Model file for the job. Use its own axes, mm. A direction names the side the tool comes from. Give positions to 0.01 mm unless a question says otherwise; leave off trailing zeros. Loops run counter-clockwise (first coordinate to the right, second up) from the corner with the lowest first, then second, coordinate; pieces in that order, holes last. Notation, with made-up numbers: M 33.5,-23 L 82.5,-23 A23 ccw 82.5,3 Z; hole C 52,-4.5 d10. An arc over 180 degrees is marked long. Answer in a Markdown table with one row per item.
```python
from build123d import *

# Parameters (mm, degrees)
BOSS_EXTRUDE1_DEPTH = 40
CUT_EXTRUDE1_REACH  = 97.146
SKETCH2_W           = 12.7
SKETCH2_H           = 36.204742391
CUT_EXTRUDE2_REACH  = 87.131
SKETCH3_W           = 56.49525371
SKETCH3_H           = 18.41246495
BOSS_EXTRUDE3_DEPTH = 2


with BuildPart() as part:
    # Sketch1 → Boss-Extrude1 (new body)
    with BuildSketch(Plane.XY):
        Polygon((-19.897004387, 33.25), (-35, 20.138954141), (-35, -20.138954141), (-19.897004387, -33.25), (19.897004387, -33.25), (35, -20.138954141), (35, 20.138954141), (19.897004387, 33.25), align=None)
        Polygon((19.15, 31.25), (33, 19.226690863), (33, -19.226690863), (19.15, -31.25), (-19.15, -31.25), (-33, -19.226690863), (-33, 19.226690863), (-19.15, 31.25), align=None, mode=Mode.SUBTRACT)
    extrude(amount=BOSS_EXTRUDE1_DEPTH)

    # Sketch2 → Cut-Extrude1 (cut, up to next)
    with BuildSketch(Plane(origin=(25.010799593, -28.810668547, 0), x_dir=(0.7551497806531032, 0.6555522929405175, 0), z_dir=(0.6555522929405175, -0.7551497806531032, 0)), mode=Mode.PRIVATE) as cut_extrude1_sk1:
        with Locations((6.878104758, 33.102371196)):
            Rectangle(SKETCH2_W, SKETCH2_H)
    cut_extrude1_tool1 = extrude(cut_extrude1_sk1.sketch, amount=-CUT_EXTRUDE1_REACH, mode=Mode.PRIVATE) & part.part
    cut_extrude1 = cut_extrude1_tool1.solids().sort_by_distance((30.204799, -24.301711, 33.102371))[0]
    add(cut_extrude1, mode=Mode.SUBTRACT)

    # Mirror1: Cut-Extrude1 across plane
    add(cut_extrude1.mirror(Plane(origin=(0, 0, 0), x_dir=(0, 0, 1), z_dir=(1, 0, 0))), mode=Mode.SUBTRACT)

    # Sketch3 → Cut-Extrude2 (cut, up to next)
    with BuildSketch(Plane.XZ.offset(33.25), mode=Mode.PRIVATE) as cut_extrude2_sk1:
        with Locations((-0.191025239, 37.206232475)):
            Rectangle(SKETCH3_W, SKETCH3_H)
    cut_extrude2_tool1 = extrude(cut_extrude2_sk1.sketch, amount=-CUT_EXTRUDE2_REACH, mode=Mode.PRIVATE) & part.part
    add(cut_extrude2_tool1.solids().sort_by_distance((-0.191025, -33.25, 37.206232))[0], mode=Mode.SUBTRACT)

    # Sketch4 → Boss-Extrude3 (add)
    with BuildSketch(Plane.XY):
        Polygon((19.15, 31.25), (33, 19.226690863), (33, -19.226690863), (19.15, -31.25), (-19.15, -31.25), (-33, -19.226690863), (-33, 19.226690863), (-19.15, 31.25), align=None)
    extrude(amount=BOSS_EXTRUDE3_DEPTH)


solid = part.part
```
Q1. Probe probe 1 along Y at (x, z) = (-13, 18.5); probe 2 along X at (y, z) = (11, 37.5); probe 3 along Z at (x, y) = (19, 17). List the from-to ranges inside material, lowest first.
Reported:
| item | result |
|---|---|
| probe 1 | -33.25 to -31.25, 31.25 to 33.25 |
| probe 2 | -35 to -33, 33 to 35 |
| probe 3 | 0 to 2 |
Q2. 3-axis set-ups, long thin cutter, end or side, ignore diameter. For faces 4 (the face through (-26.172, 25.154, 20.734)), 5 (the face through (25.665, -28.243, 10.693)): which of +Z, -Z, +X, -X, +Y, -Y reach the whole face in a straight line?
Reported:
| item | result |
|---|---|
| face 4 | +Z |
| face 5 | +Z, -Z, +X, -Y |
Q3. Saw through at B-B (y = 15.5). Give the cut face in (x, z), and give its area (3 significant figures).
Reported:
| item | result |
|---|---|
| outline | M -35,0 L 35,0 L 35,40 L 33,40 L 33,2 L -33,2 L -33,40 L -35,40 Z |
| area | 292 mm² |
Q4. Drop flat-ended pins along their axis: pin 1 (5 mm diameter, centred on x = 12, y = -31.5, fed in from +Z); pin 2 (5 mm diameter, centred on x = -5.5, y = 0, fed in from +Z); pin 3 (1 mm diameter, centred on x = -5, z = 32.5, fed in from -Y). Give the stop position or say it passes through.
Reported:
| item | result |
|---|---|
| pin 1 | z = 28 |
| pin 2 | z = 2 |
| pin 3 | y = 31.25 |
Q5. Mould opens along Y. For faces 1 (the face through (0, -32, 28)), 2 (the face through (0, -31.25, 15)), 3 (the face through (-25.876, -28.059, 10.693)) say: released by +Y, released by -Y, zero draft, split by the parting line, or undercut.
Reported:
| item | result |
|---|---|
| face 1 | zero draft |
| face 2 | undercut |
| face 3 | released by -Y |
Q6. Saw through at C-C (x = 2.5). Give the cut face in (y, z).
Reported:
| item | result |
|---|---|
| outline | M -33.25,0 L 33.25,0 L 33.25,40 L 31.25,40 L 31.25,2 L -31.25,2 L -31.25,28 L -33.25,28 Z |
Q7. Saw through at A-A (z = 17). Give the cut face in (x, y).
Reported:
| item | result |
|---|---|
| outline | M -35,-20.14 L -33,-17.84 L -33,19.23 L -19.15,31.25 L 19.15,31.25 L 33,19.23 L 33,-17.84 L 35,-20.14 L 35,20.14 L 19.9,33.25 L -19.9,33.25 L -35,20.14 Z; M -25.41,-28.46 L -19.9,-33.25 L 19.9,-33.25 L 25.41,-28.46 L 24.1,-26.95 L 19.15,-31.25 L -19.15,-31.25 L -24.1,-26.95 Z |
